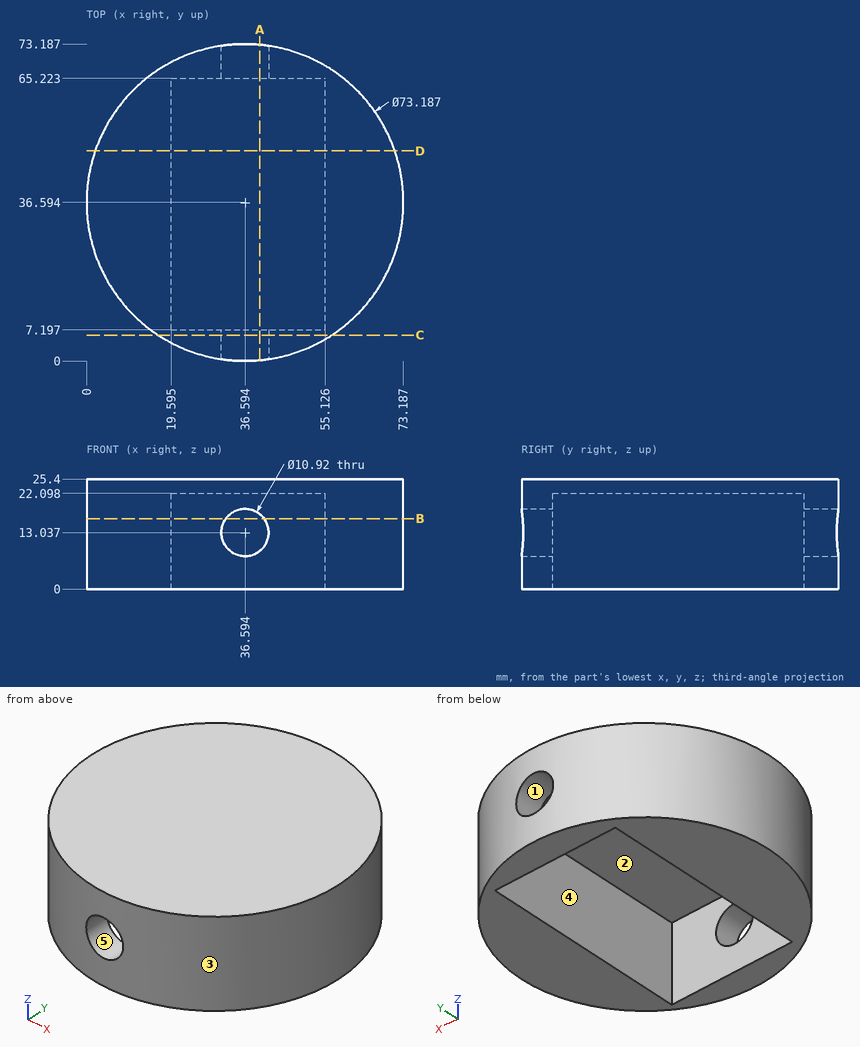
Job drawing, mm, ordinate dimensions from the low corner. One solid piece. A direction names the side the tool comes from. Give positions to 0.01 mm unless a question says otherwise; leave off trailing zeros. Loops run counter-clockwise (first coordinate to the right, second up) from the corner with the lowest first, then second, coordinate; pieces in that order, holes last. Notation, with made-up numbers: (27.25, 52) -> (32.25, 52) arc R24 ccw to (32.25, 83) -> close; hole circle Ø4 at (82, 81.5). An arc over 180 degrees is marked (long way). Use a Markdown table: item, result. Add a question column.
(1) Mould opens along Y. For the marked faces 1, 2 and 3 say: +Y half, -Y half, draft (parallel to the pull), parting line (faces both ways), or undercut.
(2) Wall check: line 1 along X through (y, z) = (35.5, 2.75) (1 decimal); line 2 along Z through (x, y) = (24, 9); line 3 along X through (y, z) = (25, 9.25) (1 decimal). Give the ranges that are in metal, low to high.
(3) Slice it at D-D on y = 48.5. List the corners of the cut face in (x, z) (1 decimal).
(4) Slice it at A-A on x = 40. List the corners of the cut face in (y, z).
(5) Drop flat-ended pins along their axis: pin 1 Ø12 at (x, z) = (8.5, 19.5) entering from +Y (1 decimal); pin 2 Ø6.5 at (y, z) = (24.5, 6) entering from +X; pin 3 Ø12 at (y, z) = (59.5, 3) entering from -X; pin 4 Ø10 at (x, y) = (24.5, 25.5) entering from -Z. Give the stop position or say it passes through.
(6) Tool access for the marked faces 4 and 5: list every direction of +Z, -Z, +X, -X, +Y, -Y with a clear straight run to the whole face (end or side of a thin tool).
(7) Slice it at C-C on y = 6. List the corners of the cut face in (x, z) (1 decimal).
(8) Slice it at B-B on z = 16.25. List the corners of the cut face in (x, y) (1 decimal).
Filled sheet:
| question | item | result |
|---|---|---|
| 1 | face 1 | draft |
| 1 | face 2 | undercut |
| 1 | face 3 | parting line |
| 2 | line 1 | 0 to 19.6, 55.1 to 73.2 |
| 2 | line 2 | 22.1 to 25.4 |
| 2 | line 3 | 1.9 to 19.6, 55.1 to 71.3 |
| 3 | outline | (2, 0) -> (19.6, 0) -> (19.6, 22.1) -> (55.1, 22.1) -> (55.1, 0) -> (71.2, 0) -> (71.2, 25.4) -> (2, 25.4) -> close |
| 4 | outline | (0.16, 0) -> (7.2, 0) -> (7.2, 8.77) -> (0.16, 8.77) -> close; (0.16, 17.3) -> (7.2, 17.3) -> (7.2, 22.1) -> (65.22, 22.1) -> (65.22, 17.3) -> (73.03, 17.3) -> (73.03, 25.4) -> (0.16, 25.4) -> close; (65.22, 0) -> (73.03, 0) -> (73.03, 8.77) -> (65.22, 8.77) -> close |
| 5 | pin 1 | y = 65.8 |
| 5 | pin 2 | x = 72.1 |
| 5 | pin 3 | x = 4.14 |
| 5 | pin 4 | z = 0 |
| 6 | face 4 | -Z |
| 6 | face 5 | +Y, -Y |
| 7 | outline | (16.5, 0) -> (56.7, 0) -> (56.7, 25.4) -> (16.5, 25.4) -> close; hole circle Ø10.9 at (36.6, 13) |
| 8 | outline | (19.6, 7.2) -> (19.6, 65.2) -> (32.2, 65.2) -> (32.2, 72.9) arc R36.6 ccw to (32.2, 0.3) -> (32.2, 7.2) -> close; (41, 0.3) arc R36.6 ccw to (41, 72.9) -> (41, 65.2) -> (55.1, 65.2) -> (55.1, 7.2) -> (41, 7.2) -> close |
